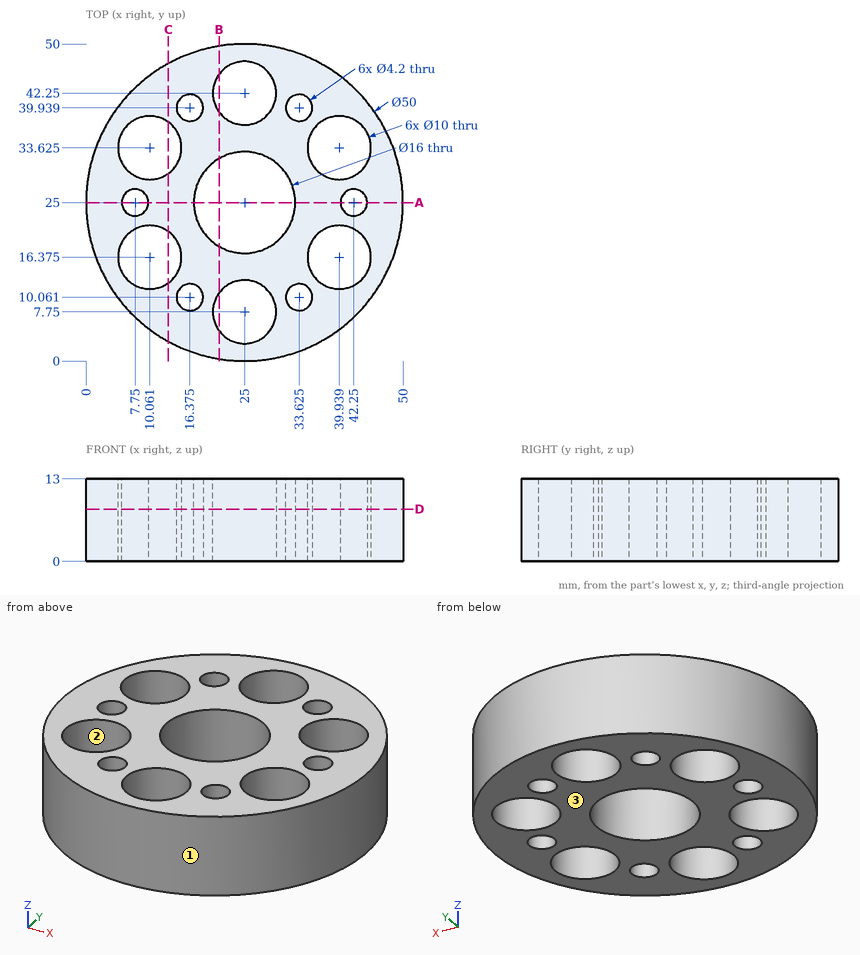
Part print with two shaded views. Sizes in mm from the minimum x, y, z corner. Coordinates: 2 decimals unless noted, no trailing zeros. Write each loop counter-clockwise with the first axis right and the second up, starting at its lowest first coordinate (ties: lowest second). Pieces come first, ordered by that corner, then holes. Notation, with made-up numbers: (20.25, 87) -> (26.25, 87) arc R32 cw to (26.25, 124) -> close; hole circle Ø9 at (4.5, 27.5). An arc over 180 degrees is marked (long way). Return JSON: item names as keys, results as strings. Group by question number.
Q1. Pull direction Y, two halves, no side cores. Call the marked faces 1, 2 and 3: released by +Y, released by -Y, zero draft, split by the parting line, or undercut.
Q2. Drill centre lines: line 1 (Y direction, x = 25, z = 3); line 2 (Y direction, x = 16.5, z = 7.25) (1 decimal); line 3 (Y direction, x = 23, z = 10). Where is each one in solid material? Low to high.
Q3. Cut at B-B, the plane x = 21. Give the cut face in (y, z), then the cut area to 4 significant figures.
Q4. Cut at D-D, the plane z = 8.25. State how many separate pieces and enclosed holes the cut face has, then the cut area to 3 significant figures.
Q5. Cut at A-A, the plane y = 25. Give the cut face in (x, z), then the cut area to 3 significant figures.
Q6. Flat gauge pin, fed straight in: pin 1 (4 mm diameter, centred on y = 7.5, z = 5.5, fed in from +X) (3 decimals). Where does the tip first touch, or does it go through?
Q7. Cut at C-C, the plane x = 13. Give the cut face in (y, z).
Returned:
{
 "1": {"face 1": "split by the parting line", "face 2": "undercut", "face 3": "zero draft"},
 "2": {"line 1": "y = 0 to 2.75, 12.75 to 17, 33 to 37.25, 47.25 to 50", "line 2": "y = 1.5 to 8, 12.2 to 37.8, 42 to 48.5", "line 3": "y = 0.08 to 3.17, 12.33 to 17.25, 32.75 to 37.67, 46.83 to 49.92"},
 "3": {"outline": "(0.32, 0) -> (4.75, 0) -> (4.75, 13) -> (0.32, 13) -> close; (10.75, 0) -> (18.07, 0) -> (18.07, 13) -> (10.75, 13) -> close; (31.93, 0) -> (39.25, 0) -> (39.25, 13) -> (31.93, 13) -> close; (45.25, 0) -> (49.68, 0) -> (49.68, 13) -> (45.25, 13) -> close", "area": "305.5 mm2"},
 "4": {"separate pieces": "1", "enclosed holes": "13", "area": "1,210 mm2"},
 "5": {"outline": "(0, 0) -> (5.65, 0) -> (5.65, 13) -> (0, 13) -> close; (9.85, 0) -> (17, 0) -> (17, 13) -> (9.85, 13) -> close; (33, 0) -> (40.15, 0) -> (40.15, 13) -> (33, 13) -> close; (44.35, 0) -> (50, 0) -> (50, 13) -> (44.35, 13) -> close", "area": "333 mm2"},
 "6": {"pin 1": "stops at x = 44.615"},
 "7": {"outline": "(3.07, 0) -> (12.33, 0) -> (12.33, 13) -> (3.07, 13) -> close; (20.42, 0) -> (29.58, 0) -> (29.58, 13) -> (20.42, 13) -> close; (37.67, 0) -> (46.93, 0) -> (46.93, 13) -> (37.67, 13) -> close"}
}
